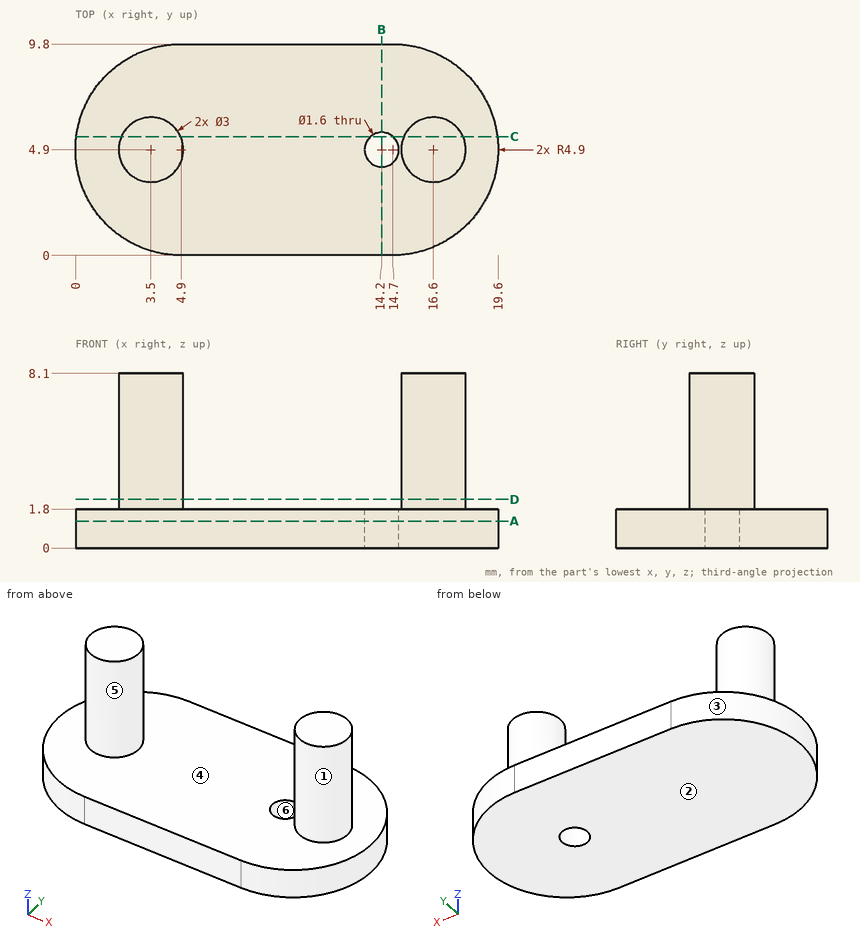
Design review of the part shown in the three views and the two pictorial views. Dimensions are in mm from the part's minimum x, y and z. A direction names the side the tool comes from. Round coordinates to 2 decimals unless told otherwise and drop trailing zeros. Loops run counter-clockwise (first coordinate to the right, second up) from the corner with the lowest first, then second, coordinate; pieces in that order, holes last. Notation, with made-up numbers: (31, -15.5) - (52, -15.5) arc R33 cw to (52, 16.5) - close; hole circle Ø4 at (33.25, -1.75). An arc over 180 degrees is marked (long way). Write each question's results on one line, items separated by ' | '. Start each with the question number.
Q1. Take a section at C-C on y = 5.5. Give the boundary of the cut face in (x, z), plus the area to 3 significant figures.
Q2. Take a section at D-D on z = 2.25. Give the boundary of the cut face in (x, y).
Q3. Wall thickness on line 1 along Y through (x, z) = (14.2, 1.2); line 2 along Z through (x, y) = (17, 6.5); line 3 along X through (y, z) = (4, 2): over which ranges is each line inside the solid? List them lowest first. Write a range as [from, to].
Q4. Tool access review of the marked faces 5 and 6: name each direction out of +Z, -Z, +X, -X, +Y, -Y from which nothing blocks a thin tool from reaching the whole face with its end or side.
Q5. Take a section at B-B on x = 14.2. Give the boundary of the cut face in (y, z).
Q6. Draft analysis for pull direction X (two halves, no side actions). For the marked faces 1, 2, 3 and 4, state which applies: pulls with the +X half, pulls with the -X half, needs draft (parallel to the pull), parting line crosses it, or undercut.
Q7. Take a section at A-A on z = 1.25. Give the boundary of the cut face in (x, y), plus the area to 3 significant figures.
Q8. Insertion check: P1, Ø2, axis at x = 12.5, y = 6.5, coming from the +Z side; P2, Ø4, axis at y = 1, z = 2, coming from the +X side; P3, Ø4, axis at x = 3.5, z = 5, coming from the +Y side; P4, Ø1, axis at y = 1.5, z = 6.5, coming from the -X side. Each pin has a flat end and moves straight along its axis. Give the tip position at first contact, or say it passes through.
Data:
1) outline: (0.04, 0) - (13.67, 0) - (13.67, 1.8) - (4.87, 1.8) - (4.87, 8.1) - (2.13, 8.1) - (2.13, 1.8) - (0.04, 1.8) - close; (14.73, 0) - (19.56, 0) - (19.56, 1.8) - (17.97, 1.8) - (17.97, 8.1) - (15.23, 8.1) - (15.23, 1.8) - (14.73, 1.8) - close | area: 67.9 mm²
2) outline: circle Ø3 at (3.5, 4.9); circle Ø3 at (16.6, 4.9)
3) line 1: y = [0, 4.1], [5.7, 9.8] | line 2: z = [0, 1.8] | line 3: x = [2.3, 4.7], [15.4, 17.8]
4) face 5: +Z | face 6: +Z, -Z
5) outline: (0, 0) - (4.1, 0) - (4.1, 1.8) - (0, 1.8) - close; (5.7, 0) - (9.8, 0) - (9.8, 1.8) - (5.7, 1.8) - close
6) face 1: undercut | face 2: needs draft | face 3: pulls with the -X half | face 4: undercut
7) outline: (4.9, 0) - (14.7, 0) arc R4.9 ccw to (14.7, 9.8) - (4.9, 9.8) arc R4.9 ccw to start; hole circle Ø1.6 at (14.2, 4.9) | area: 169 mm²
8) P1: stops at z = 1.8 | P2: stops at x = 19.21 | P3: stops at y = 6.4 | P4: passes through
